from build123d import *

# Parameters (mm, degrees)
F0_W     = 156.3
F0_H     = 75.340103
F0_R     = 6.5
F0_R_2   = 6.25
F0_R_3   = 6
F0_R_4   = 5.75
F0_R_5   = 5.5
F0_R_6   = 5.25
F0_R_7   = 6.75
F0_R_8   = 7
F0_R_9   = 7.25
F0_R_10  = 7.5
F0_R_11  = 7.75
F0_R_12  = 5
F0_R_13  = 4.75
F0_R_14  = 4.5
F0_R_15  = 4.25
F0_R_16  = 4
F0_R_17  = 3.5
F0_R_18  = 3.75
F0_R_19  = 8
F0_R_20  = 8.25
F0_R_21  = 8.5
F0_R_22  = 8.75
F0_R_23  = 10.5
F0_R_24  = 10.25
F0_R_25  = 10
F0_R_26  = 10.75
F0_R_27  = 11
F0_R_28  = 11.25
F0_R_29  = 9.75
F0_R_30  = 9.5
F0_R_31  = 9.25
F0_R_32  = 9
F0_R_33  = 11.5
F0_R_34  = 11.75
F0_R_35  = 12
F1_DEPTH = 3


with BuildPart() as f1:
    # F0 (on Top) → F1 (new body)
    with BuildSketch(Plane.XY):
        with Locations((-78.15, -37.670051)):
            Rectangle(F0_W, F0_H)
        with Locations((-143.85, -67.640103)):
            Circle(F0_R, mode=Mode.SUBTRACT)
        with Locations((-129.9, -67.890103)):
            Circle(F0_R_2, mode=Mode.SUBTRACT)
        with Locations((-116.45, -68.140103)):
            Circle(F0_R_3, mode=Mode.SUBTRACT)
        with Locations((-103.5, -68.390103)):
            Circle(F0_R_4, mode=Mode.SUBTRACT)
        with Locations((-91.05, -68.640103)):
            Circle(F0_R_5, mode=Mode.SUBTRACT)
        with Locations((-79.1, -68.890103)):
            Circle(F0_R_6, mode=Mode.SUBTRACT)
        with Locations((-145.95, -52.934465)):
            Circle(F0_R_7, mode=Mode.SUBTRACT)
        with Locations((-131, -53.184465)):
            Circle(F0_R_8, mode=Mode.SUBTRACT)
        with Locations((-115.55, -53.434465)):
            Circle(F0_R_9, mode=Mode.SUBTRACT)
        with Locations((-99.6, -53.684465)):
            Circle(F0_R_10, mode=Mode.SUBTRACT)
        with Locations((-83.15, -53.934465)):
            Circle(F0_R_11, mode=Mode.SUBTRACT)
        with Locations((-67.65, -69.140103)):
            Circle(F0_R_12, mode=Mode.SUBTRACT)
        with Locations((-56.7, -69.390103)):
            Circle(F0_R_13, mode=Mode.SUBTRACT)
        with Locations((-46.25, -69.640103)):
            Circle(F0_R_14, mode=Mode.SUBTRACT)
        with Locations((-36.3, -69.890103)):
            Circle(F0_R_15, mode=Mode.SUBTRACT)
        with Locations((-26.85, -70.140103)):
            Circle(F0_R_16, mode=Mode.SUBTRACT)
        with Locations((-9.45, -70.640103)):
            Circle(F0_R_17, mode=Mode.SUBTRACT)
        with Locations((-17.9, -70.390103)):
            Circle(F0_R_18, mode=Mode.SUBTRACT)
        with Locations((-66.2, -54.184465)):
            Circle(F0_R_19, mode=Mode.SUBTRACT)
        with Locations((-48.75, -54.434465)):
            Circle(F0_R_20, mode=Mode.SUBTRACT)
        with Locations((-30.8, -54.684465)):
            Circle(F0_R_21, mode=Mode.SUBTRACT)
        with Locations((-12.35, -54.934465)):
            Circle(F0_R_22, mode=Mode.SUBTRACT)
        with Locations((-139.5, -34.447785)):
            Circle(F0_R_23, mode=Mode.SUBTRACT)
        with Locations((-117.55, -34.734465)):
            Circle(F0_R_24, mode=Mode.SUBTRACT)
        with Locations((-96.1, -34.984465)):
            Circle(F0_R_25, mode=Mode.SUBTRACT)
        with Locations((-138.65, -11.95)):
            Circle(F0_R_26, mode=Mode.SUBTRACT)
        with Locations((-115.7, -12.2)):
            Circle(F0_R_27, mode=Mode.SUBTRACT)
        with Locations((-92.25, -12.45)):
            Circle(F0_R_28, mode=Mode.SUBTRACT)
        with Locations((-75.15, -35.234465)):
            Circle(F0_R_29, mode=Mode.SUBTRACT)
        with Locations((-54.7, -35.484465)):
            Circle(F0_R_30, mode=Mode.SUBTRACT)
        with Locations((-34.75, -35.734465)):
            Circle(F0_R_31, mode=Mode.SUBTRACT)
        with Locations((-15.3, -35.984465)):
            Circle(F0_R_32, mode=Mode.SUBTRACT)
        with Locations((-68.3, -12.7)):
            Circle(F0_R_33, mode=Mode.SUBTRACT)
        with Locations((-43.85, -12.95)):
            Circle(F0_R_34, mode=Mode.SUBTRACT)
        with Locations((-18.9, -13.2)):
            Circle(F0_R_35, mode=Mode.SUBTRACT)
    extrude(amount=F1_DEPTH)


solid = f1.part
CAD build for the part. Positions are in the model's coordinates, mm. Give positions to 0.01 mm unless a question says otherwise; leave off trailing zeros. Write each loop counter-clockwise with the first axis right and the second up, starting at its lowest first coordinate (ties: lowest second). Pieces come first, ordered by that corner, then holes. Notation, with made-up numbers: (75, -19) - (92, -19) arc R16 ccw to (92, -8) - close; hole circle Ø1 at (5.5, 43.5). An arc over 180 degrees is marked (long way). Answer as CSV lines item,"result".
Q1. Band-saw the part on A-A (x = -36.3). Give the cut face in (y, z).
Result set:
outline,"(-75.34, 0) - (-74.14, 0) - (-74.14, 3) - (-75.34, 3) - close; (-65.64, 0) - (-61.17, 0) - (-61.17, 3) - (-65.64, 3) - close; (-48.2, 0) - (-44.85, 0) - (-44.85, 3) - (-48.2, 3) - close; (-26.62, 0) - (-21.95, 0) - (-21.95, 3) - (-26.62, 3) - close; (-3.95, 0) - (0, 0) - (0, 3) - (-3.95, 3) - close"
Q2. Band-saw the part on C-C (x = -18.9). Give the cut face in (y, z).
Result set:
outline,"(-75.34, 0) - (-74, 0) - (-74, 3) - (-75.34, 3) - close; (-66.78, 0) - (-60.74, 0) - (-60.74, 3) - (-66.78, 3) - close; (-49.13, 0) - (-44.23, 0) - (-44.23, 3) - (-49.13, 3) - close; (-27.74, 0) - (-25.2, 0) - (-25.2, 3) - (-27.74, 3) - close; (-1.2, 0) - (0, 0) - (0, 3) - (-1.2, 3) - close"
Q3. Drill centre lines: line 1 (Y direction, x = -36.5, z = 1.7); line 2 (Y direction, x = -20, z = 2.65); line 3 (Y direction, x = -13, z = 1.55). Where is each one in solid material? Low to high. Write a range as from..to.
Result set:
line 1,"-75.34..-74.14, -65.64..-60.99, -48.38..-44.82, -26.65..-22.12, -3.78..0"
line 2,"-75.34..-73.5, -67.28..-59.18, -50.69..-43.66, -28.31..-25.15, -1.25..0"
line 3,"-75.34..-63.66, -46.21..-44.69, -27.28..-23.65, -2.75..0"
Q4. Band-saw the part on B-B (y = -40). State how many separate pieces and enclosed holes the cut face has, and give its area (3 significant figures).
Result set:
separate pieces,"8"
enclosed holes,"0"
area,"112 mm²"
Q5. Flat gauge pin, fed straight in: pin 1 Ø8 at (x, y) = (-143.85, -67.64) entering from -Z. Where does the tip first touch, or does it go through?
Result set:
pin 1,"through"
